Can you work these out from the drawing? Everything is in mm from the part's minimum corner. Round coordinates to 2 decimals unless told otherwise and drop trailing zeros. Order: outer loops, then holes, each group sorted by start corner. A loop starts at its lowest first (then second) coordinate and runs counter-clockwise, first axis right, second up. Notation, with made-up numbers: (44, 27) -> (90, 27) arc R26 cw to (90, 64) -> close; hole circle Ø6 at (59.25, 68.5). An arc over 180 degrees is marked (long way). One line per item, written item: value.
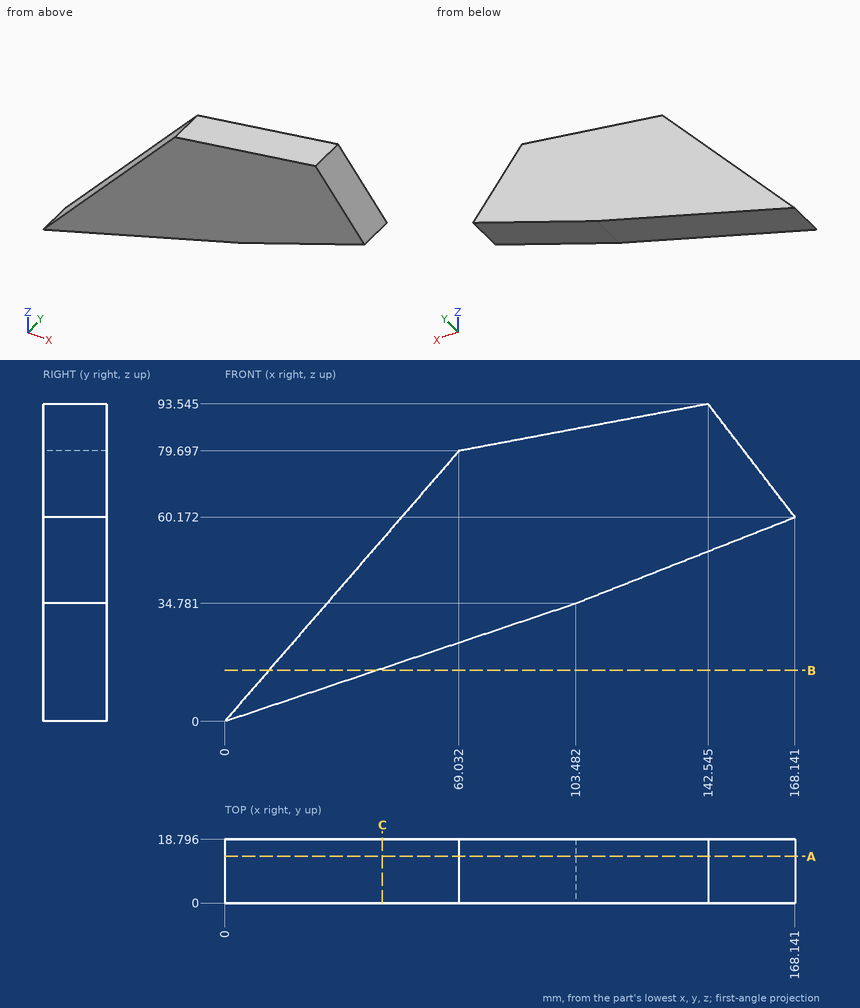
Q1. I want a section at A-A on y = 13.75. List the corners of the cut face in (x, z) for me (1 decimal), plus the area to 3 significant figures.
Answers below:
outline: (0, 0) -> (103.5, 34.8) -> (168.1, 60.2) -> (142.5, 93.5) -> (69, 79.7) -> close
area: 6,220 mm^2
Q2. Will these pins go through, and if not, where does the flat tip stop? pin 1 Ø5 at (y, z) = (6.5, 67.5) entering from +X; pin 2 Ø10 at (x, y) = (97, 14.5) entering from +Z; pin 3 Ø6 at (x, z) = (41, 50.5) entering from -Y; pin 4 Ø5 at (x, y) = (60.5, 11.5) entering from -Z (1 decimal).
Answers below:
pin 1: x = 164.44
pin 2: z = 85.91
pin 3: y = 0
pin 4: z = 19.5
Q3. I want a section at B-B on z = 15. List the corners of the cut face in (x, y) for me.
Answers below:
outline: (12.99, 0) -> (44.63, 0) -> (44.63, 18.8) -> (12.99, 18.8) -> close
Q4. I want a section at C-C on x = 46.5. List the corners of the cut face in (y, z) for me (1 decimal), plus the area to 3 significant figures.
Answers below:
outline: (0, 15.6) -> (18.8, 15.6) -> (18.8, 53.7) -> (0, 53.7) -> close
area: 715 mm^2
Q5. Please list where these lines run through material, in increasing order: line 1 along Z through (x, y) = (131, 4.75); line 2 along X through (y, z) = (12.5, 71) (1 decimal); line 3 along Z through (x, y) = (84, 1.75).
Answers below:
line 1: 45.59 to 91.37
line 2: 61.5 to 159.8
line 3: 28.23 to 82.52
